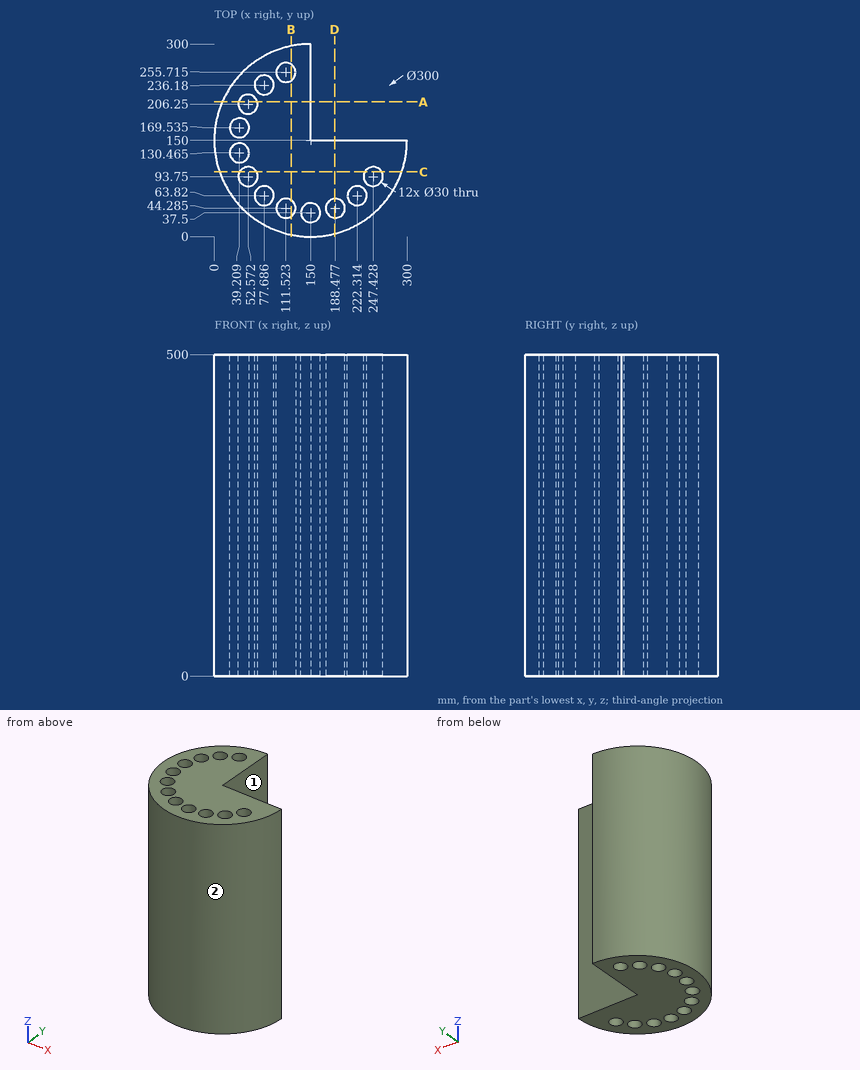
Source: three-view drawing plus pictorial views. Frame: mm from the lowest corner of the part. A direction names the side the tool comes from. Round coordinates to 2 decimals unless told otherwise and drop trailing zeros. Loops run counter-clockwise (first coordinate to the right, second up) from the corner with the lowest first, then second, coordinate; pieces in that order, holes last.
Item 1: Section C-C, the plane y = 101. Output: boundary loops of the cut face in (x, z).
Checked values:
outline: (8.23, 0) - (39.44, 0) - (39.44, 500) - (8.23, 500) - close; (65.7, 0) - (234.3, 0) - (234.3, 500) - (65.7, 500) - close; (260.56, 0) - (291.77, 0) - (291.77, 500) - (260.56, 500) - close
Item 2: Contact query for flat-ended pins moving along their axis: P1, Ø24, axis at x = 188.48, y = 44.28, coming from the -Z side; P2, Ø1, axis at y = 63, z = 445, coming from the -X side; P3, Ø4, axis at x = 88.5, z = 288, coming from the -Y side (1 decimal); P4, Ø5, axis at y = 211, z = 166.5, coming from the -X side. Output: stop coordinate, or through.
Checked values:
P1: passes through
P2: stops at x = 27.45
P3: stops at y = 12.3
P4: stops at x = 11.88
Item 3: Section B-B, the plane x = 119.5. Output: boundary loops of the cut face in (y, z).
Checked values:
outline: (3.13, 0) - (31.58, 0) - (31.58, 500) - (3.13, 500) - close; (56.99, 0) - (243.01, 0) - (243.01, 500) - (56.99, 500) - close; (268.42, 0) - (296.87, 0) - (296.87, 500) - (268.42, 500) - close
Item 4: Section D-D, the plane x = 187.5. Output: boundary loops of the cut face in (y, z), plus the area to 4 significant figures.
Checked values:
outline: (4.76, 0) - (29.32, 0) - (29.32, 500) - (4.76, 500) - close; (59.25, 0) - (150, 0) - (150, 500) - (59.25, 500) - close
area: 57,650 mm2
Item 5: Reachability of the marked faces 1 and 2 from +Z, -Z, +X, -X, +Y, -Y: full face, straight path, thin tool, end or side. Return the list, or none.
Checked values:
face 1: +Z, -Z, +X, +Y
face 2: +Z, -Z
Item 6: Line query: L1, parallel to X at y = 60.5, z = 284 (1 decimal); L2, parallel to Y at x = 28, z = 223 (1 decimal); L3, parallel to Y at x = 100, z = 154.5. Output: solid intervals per line, ascending.
Checked values:
L1: x = 29.6 to 63.1, 92.3 to 207.7, 236.9 to 270.4
L2: y = 62.7 to 120.5, 140.4 to 159.6, 179.5 to 237.3
L3: y = 8.58 to 34.68, 53.89 to 246.11, 265.32 to 291.42
Item 7: Section A-A, the plane y = 210. Output: boundary loops of the cut face in (x, z) (1 decimal).
Checked values:
outline: (12.5, 0) - (38, 0) - (38, 500) - (12.5, 500) - close; (67.1, 0) - (150, 0) - (150, 500) - (67.1, 500) - close
